Can you work these out from the model? Positions are in its coordinate system, mm. Face numbers are marked on the shaded views. A direction names the side the tool comes from. Round coordinates to 2 decimals unless told otherwise and drop trailing zeros. Order: outer loops, then holes, each group sorted by start corner. A loop starts at its lowest first (then second) coordinate and runs counter-clockwise, first axis right, second up. Notation, with made-up numbers: (70.25, -18.75) - (118.25, -18.75) arc R24 cw to (118.25, 9.25) - close; hole circle Ø9 at (66, 35). An arc over 180 degrees is marked (long way). Write item = value, one per line.
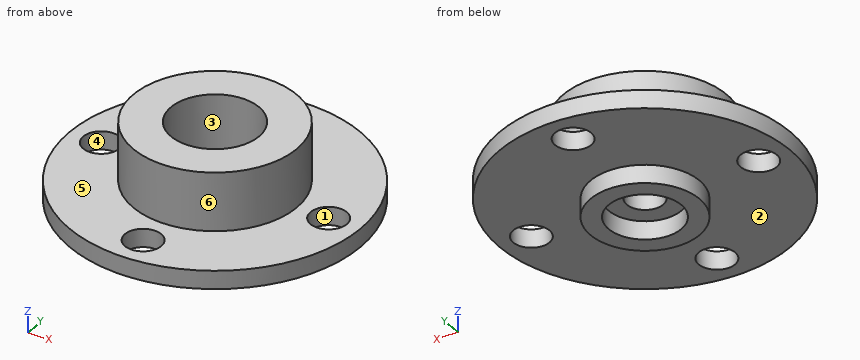
from build123d import *

# Parameters (mm, degrees)
SKETCH1_R           = 4.5
SKETCH1_R_2         = 2.425
BOSS_EXTRUDE1_DEPTH = 3.2
SKETCH1_3_R         = 8
SKETCH1_3_R_2       = 1
BOSS_EXTRUDE2_DEPTH = 1
SKETCH2_R           = 3
SKETCH2_R_2         = 2
BOSS_EXTRUDE3_DEPTH = 1


with BuildPart() as part:
    # Sketch1 → Boss-Extrude1 (new body)
    with BuildSketch(Plane.XY):
        Circle(SKETCH1_R)
        Circle(SKETCH1_R_2, mode=Mode.SUBTRACT)
    extrude(amount=BOSS_EXTRUDE1_DEPTH)

    # Sketch1<3> → Boss-Extrude2 (add)
    with BuildSketch(Plane.XY):
        Circle(SKETCH1_3_R)
        with Locations((6.25, 0)):
            Circle(SKETCH1_3_R_2, mode=Mode.SUBTRACT)
        with Locations((0, -6.25)):
            Circle(SKETCH1_3_R_2, mode=Mode.SUBTRACT)
        with Locations((-6.25, 0)):
            Circle(SKETCH1_3_R_2, mode=Mode.SUBTRACT)
        with Locations((0, 6.25)):
            Circle(SKETCH1_3_R_2, mode=Mode.SUBTRACT)
        Circle(SKETCH1_3_R_2, mode=Mode.SUBTRACT)
    extrude(amount=-BOSS_EXTRUDE2_DEPTH)

    # Sketch2 → Boss-Extrude3 (add)
    with BuildSketch(Plane(origin=(0, 0, -1), x_dir=(-1, 0, 0), z_dir=(0, 0, -1))):
        Circle(SKETCH2_R)
        Circle(SKETCH2_R_2, mode=Mode.SUBTRACT)
    extrude(amount=BOSS_EXTRUDE3_DEPTH)


solid = part.part
(1) If we section it at B-B (y = -5.5): Write out the boundary of the cut face in (x, z), plus the area to 3 significant figures.
Computed:
outline = (-5.81, -1) - (-0.66, -1) - (-0.66, 0) - (-5.81, 0) - close; (0.66, -1) - (5.81, -1) - (5.81, 0) - (0.66, 0) - close
area = 10.3 mm^2
(2) Thinking about a two-plate mould opening in X: for the marked faces 4, 5 and 6, which applies, +X half, -X half, draft (parallel to the pull), parting line (faces both ways), or undercut?
Computed:
face_4 = undercut
face_5 = draft
face_6 = parting line
(3) Will these pins go through, and if not, where does the flat tip stop? P1, Ø1.2, axis at x = -0.5, y = 1, coming from the -Z side; P2, Ø1, axis at x = 4, y = -3.5, coming from the +Z side; P3, Ø2, axis at y = 3.5, z = -1, coming from the -X side; P4, Ø8, axis at x = -1.5, y = 0.5, coming from the -Z side.
Computed:
P1 = -1
P2 = 0
P3 = -7.6
P4 = -2
(4) If I drill on line 1 (Y direction, x = 0, z = -0.7); line 2 (Z direction, x = 0.5, y = -3.5); line 3 (Z direction, x = 1.25, y = 5.5), over which ranges is the centre line in solid material (lowest first)? Write a range as from..to.
Computed:
line_1 = -8..-7.25, -5.25..-1, 1..5.25, 7.25..8
line_2 = -1..3.2
line_3 = -1..0
(5) If we section it at C-C (z = -0.3): Write out the boundary of the cut face in (x, y), plus the area to 3 significant figures.
Computed:
outline = circle Ø16 at (0, 0); hole circle Ø2 at (-6.25, 0); hole circle Ø2 at (0, -6.25); hole circle Ø2 at (0, 0); hole circle Ø2 at (0, 6.25); hole circle Ø2 at (6.25, 0)
area = 185 mm^2
(6) If we section it at A-A (x = 0): State how many separate pieces and enclosed holes the cut face has, plus the area to 3 significant figures.
Computed:
separate_pieces = 4
enclosed_holes = 0
area = 25.3 mm^2
(7) On a 3-axis mill with a long thin cutter (end or side, diameter ignored), from which of +Z, -Z, +X, -X, +Y, -Y can I reach the whole of each face in a straight line? I mean the marked faces 1, 2 and 3. Say none if no direction works.
Computed:
face_1 = +Z, -Z
face_2 = -Z
face_3 = +Z
